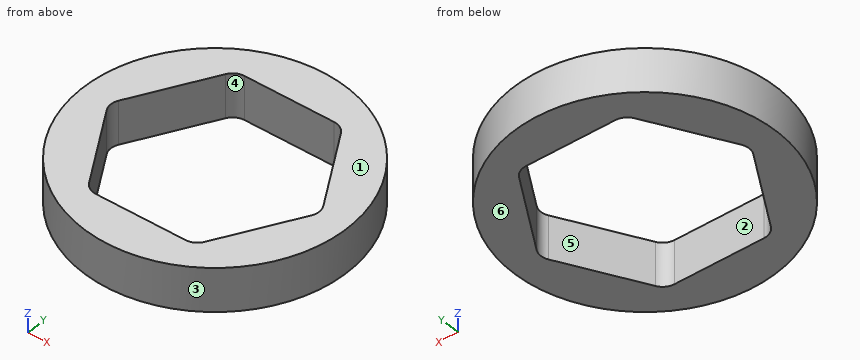
from build123d import *

# Parameters (mm, degrees)
SKETCH1_R           = 9
BOSS_EXTRUDE1_DEPTH = 3


with BuildPart() as part:
    # Sketch1 → Boss-Extrude1 (new body)
    with BuildSketch(Plane.XY.offset(3)):
        with Locations(Location((0, 0, 0), (0, 0, 180))):
            Circle(SKETCH1_R)
        with BuildLine():
            Line((-3.0022214, 6.2), (3.0022214, 6.2))
            ThreePointArc((3.0022214, 6.2), (3.5022214, 6.066025404), (3.868246804, 5.7))
            Line((3.868246804, 5.7), (6.870468203, 0.5))
            ThreePointArc((6.870468203, 0.5), (7.0044428, 0), (6.870468203, -0.5))
            Line((6.870468203, -0.5), (3.868246804, -5.7))
            ThreePointArc((3.868246804, -5.7), (3.5022214, -6.066025404), (3.0022214, -6.2))
            Line((3.0022214, -6.2), (-3.0022214, -6.2))
            ThreePointArc((-3.0022214, -6.2), (-3.5022214, -6.066025404), (-3.868246804, -5.7))
            Line((-3.868246804, -5.7), (-6.870468203, -0.5))
            ThreePointArc((-6.870468203, -0.5), (-7.0044428, 0), (-6.870468203, 0.5))
            Line((-6.870468203, 0.5), (-3.868246804, 5.7))
            ThreePointArc((-3.868246804, 5.7), (-3.5022214, 6.066025404), (-3.0022214, 6.2))
        make_face(mode=Mode.SUBTRACT)
    extrude(amount=-BOSS_EXTRUDE1_DEPTH)


solid = part.part
Could you check a few things on this model? Use its own coordinates, in mm. Face numbers are marked on the shaded views. A direction names the side the tool comes from. Coordinates: 2 decimals unless noted, no trailing zeros. Order: outer loops, then holes, each group sorted by start corner. A loop starts at its lowest first (then second) coordinate and runs counter-clockwise, first axis right, second up. Notation, with made-up numbers: (74, 54) - (124, 54) arc R23 ccw to (124, 87) - close; hole circle Ø10 at (44.25, 31). An arc over 180 degrees is marked (long way). Answer in a Markdown table with one row per item. Add a question column.
(1) If we section it at B-B, the plane x = 0: Please give me the cut outline in (y, z), then the cut area to 3 significant figures.
(2) If we section it at C-C, the plane z = 0.35: Please give me the cut outline in (x, y), then the cut area to 3 significant figures.
(3) Will these pins go through, and if not, where does the flat tip stop? pin 1 (1 mm diameter, centred on x = -5.5, z = 2.5, fed in from -Y); pin 2 (0.9 mm diameter, centred on x = -1, z = 1, fed in from +Y); pin 3 (0.9 mm diameter, centred on x = -1.5, z = 1, fed in from -Y).
(4) On a 3-axis mill with a long thin cutter (end or side, diameter ignored), from which of +Z, -Z, +X, -X, +Y, -Y can I reach the whole of each face in a straight line? I mean the marked faces 1 and 2. Say none if no direction works.
(5) If we section it at A-A, the plane y = 0: Please give me the cut outline in (x, z), then the cut area to 3 significant figures.
(6) I need wall thicknesses on L1, parallel to Y at x = 0, z = 2.85; L2, parallel to Y at x = 4.75, z = 2.35; L3, parallel to X at y = 2.5, z = 0.95. Which ranges of each line are inside material? Lowest first, please.
(7) If we mould it in two halves opening along X, with no side actions, what happens to the marked faces 3, 4, 5 and 6? For each: released by +X, released by -X, zero draft, split by the parting line, or undercut.
(8) If we section it at D-D, the plane x = 7.5: Please give me the cut outline in (y, z).
Results are:
| question | item | result |
|---|---|---|
| 1 | outline | (-9, 0) - (-6.2, 0) - (-6.2, 3) - (-9, 3) - close; (6.2, 0) - (9, 0) - (9, 3) - (6.2, 3) - close |
| 1 | area | 16.8 mm2 |
| 2 | outline | circle Ø18 at (0, 0); hole (-6.87, -0.5) - (-3.87, -5.7) arc R1 ccw to (-3, -6.2) - (3, -6.2) arc R1 ccw to (3.87, -5.7) - (6.87, -0.5) arc R1 ccw to (6.87, 0.5) - (3.87, 5.7) arc R1 ccw to (3, 6.2) - (-3, 6.2) arc R1 ccw to (-3.87, 5.7) - (-6.87, 0.5) arc R1 ccw to start |
| 2 | area | 122 mm2 |
| 3 | pin 1 | stops at y = -7.48 |
| 3 | pin 2 | stops at y = 8.98 |
| 3 | pin 3 | stops at y = -8.94 |
| 4 | face 1 | +Z, +X, -X, +Y, -Y |
| 4 | face 2 | +Z, -Z |
| 5 | outline | (-9, 0) - (-7, 0) - (-7, 3) - (-9, 3) - close; (7, 0) - (9, 0) - (9, 3) - (7, 3) - close |
| 5 | area | 12.0 mm2 |
| 6 | L1 | y = -9 to -6.2, 6.2 to 9 |
| 6 | L2 | y = -7.64 to -4.17, 4.17 to 7.64 |
| 6 | L3 | x = -8.65 to -5.72, 5.72 to 8.65 |
| 7 | face 3 | split by the parting line |
| 7 | face 4 | undercut |
| 7 | face 5 | undercut |
| 7 | face 6 | zero draft |
| 8 | outline | (-4.97, 0) - (4.97, 0) - (4.97, 3) - (-4.97, 3) - close |
